Here's how the part is built. I have some questions about the finished solid (model axes, mm). A direction names the side the tool comes from. Round coordinates to 2 decimals unless told otherwise and drop trailing zeros. Order: outer loops, then holes, each group sorted by start corner. A loop starts at its lowest first (then second) coordinate and runs counter-clockwise, first axis right, second up. Notation, with made-up numbers: M 11,59.5 L 60,59.5 A27 cw 60,83.5 Z; hole C 85,-9.75 d6. An arc over 180 degrees is marked long. Write item = value, one per line. Start each with the question number.
Item 1: I want a section at D-D, the plane y = -4. List the corners of the cut face in (x, z) for me.
Item 2: We'd pull the mould along Z, two halves only. Please class faces 6 (the face through (23, -6, -13)), 7 (the face through (16.57, 6.1, 1.48)), 8 (the face through (20.76, 15.537, -7.798)): pulls with the +Z half, pulls with the -Z half, needs draft (parallel to the pull), parting line crosses it, or undercut.
Item 3: I want a section at C-C, the plane z = -8. State how many separate pieces and enclosed holes the cut face has, plus the area to 3 significant figures.
Item 4: I want a section at A-A, the plane z = -5.75. List the corners of the cut face in (x, y) for me, plus the area to 3 significant figures.
Item 5: I want a section at B-B, the plane x = 11.75. List the corners of the cut face in (y, z) for me.
Item 6: Please list where these lines run through material, in increasing order: L1, parallel to X at y = 11, z = -1; L2, parallel to Y at x = 23.35, z = -8; L3, parallel to Y at x = 25, z = -7.5.
Item 7: I'm going to push flat-ended pins straight in: P1, Ø2, axis at y = 6, z = -11.5, coming from the -X side; P2, Ø8, axis at x = 5, z = -0.5, coming from the -Y side; P3, Ø1.6, axis at x = 20.5, y = -1, coming from the +Z side; P4, Ø9.5, axis at x = 25, y = 5, coming from the -Z side. Where does each tip first touch, or does it pass through?
Item 8: For faces 1 (the face through (29.048, 5.127, -7.605)), 2 (the face through (9, 7, 0)), 3 (the face through (23, 15, -1)), 4 (the face through (23.26, 15.537, -7.798)), 5 (the face through (16.55, 3.88, 1.48)), which set-ups out of +Z, -Z, +X, -X, +Y, -Y let a thin tool reach every point of the face, with its end or its side?
```python
from build123d import *

# Parameters (mm, degrees)
SZKIC1_W                    = 30
SZKIC1_H                    = 10
DODANIE_WYCI_GNI_CIE1_DEPTH = 3
ZAOKR_GLENIE1_R             = 5
WYTNIJ_WYCI_GNI_CIE1_REACH  = 33.765
SZKIC2_W                    = 13.6
SZKIC2_H                    = 3.1
ZAOKR_GLENIE2_R             = 1.5
SZKIC3_R                    = 5
DODANIE_WYCI_GNI_CIE2_DEPTH = 15
SZKIC5_W                    = 1.5
SZKIC5_H                    = 24
DODANIE_WYCI_GNI_CIE3_DEPTH = 15
SZKIC4_R                    = 4.05
WYTNIJ_WYCI_GNI_CIE2_DEPTH  = 15
SZKIC6_W                    = 1
SZKIC6_H                    = 10.631374676
WYTNIJ_WYCI_GNI_CIE3_DEPTH  = 15
SZKIC7_R                    = 1.55
WYTNIJ_WYCI_GNI_CIE4_DEPTH  = 34.015148038
ZAOKR_GLENIE3_R             = 5
SFAZOWANIE1_SIZE            = 1


with BuildPart() as part:
    # Szkic1 → Dodanie-wyciągnięcie1 (new body)
    with BuildSketch(Plane.XY):
        with Locations((15, 5)):
            Rectangle(SZKIC1_W, SZKIC1_H)
    extrude(amount=DODANIE_WYCI_GNI_CIE1_DEPTH)

    # Zaokrąglenie1
    zaokr_glenie1_edges = [part.edges().sort_by_distance(p)[0] for p in [
        (0, 10, 1.5),
        (0, 0, 1.5),
        (30, 10, 1.5),
        (30, 0, 1.5),
    ]]
    fillet(zaokr_glenie1_edges, radius=ZAOKR_GLENIE1_R - 0.0001)  # a hair under: the kernel refuses the full size

    # Szkic2 → Wytnij-wyciągnięcie1 (cut, up to next)
    with BuildSketch(Plane.XY.offset(3), mode=Mode.PRIVATE) as wytnij_wyci_gni_cie1_sk1:
        with Locations((10.2, 5)):
            Rectangle(SZKIC2_W, SZKIC2_H)
    wytnij_wyci_gni_cie1_tool1 = extrude(wytnij_wyci_gni_cie1_sk1.sketch, amount=-WYTNIJ_WYCI_GNI_CIE1_REACH, mode=Mode.PRIVATE) & part.part
    add(wytnij_wyci_gni_cie1_tool1.solids().sort_by_distance((10.2, 5, 3))[0], mode=Mode.SUBTRACT)

    # Zaokrąglenie2
    zaokr_glenie2_edges = [part.edges().sort_by_distance(p)[0] for p in [
        (3.4, 3.45, 1.5),
        (3.4, 6.55, 1.5),
        (17, 6.55, 1.5),
        (17, 3.45, 1.5),
    ]]
    fillet(zaokr_glenie2_edges, radius=ZAOKR_GLENIE2_R)

    # Szkic3 → Dodanie-wyciągnięcie2 (add)
    with BuildSketch(Plane(origin=(0, 0, 0), x_dir=(-1, 0, 0), z_dir=(0, 0, -1))):
        with Locations((-25, 5)):
            Circle(SZKIC3_R)
    extrude(amount=DODANIE_WYCI_GNI_CIE2_DEPTH)

    # Szkic5 → Dodanie-wyciągnięcie3 (add)
    with BuildSketch(Plane(origin=(0, 0, -15), x_dir=(-1, 0, 0), z_dir=(0, 0, -1))):
        with Locations((-20.75, 5)):
            Rectangle(SZKIC5_W, SZKIC5_H)
        with Locations((-23.25, 5)):
            Rectangle(SZKIC5_W, SZKIC5_H)
    extrude(amount=-DODANIE_WYCI_GNI_CIE3_DEPTH)

    # Szkic4 → Wytnij-wyciągnięcie2 (cut)
    with BuildSketch(Plane(origin=(0, 0, -15), x_dir=(-1, 0, 0), z_dir=(0, 0, -1))):
        with Locations((-25, 5)):
            Circle(SZKIC4_R)
    extrude(amount=-WYTNIJ_WYCI_GNI_CIE2_DEPTH, mode=Mode.SUBTRACT)

    # Szkic6 → Wytnij-wyciągnięcie3 (cut)
    with BuildSketch(Plane(origin=(0, 0, -15), x_dir=(-1, 0, 0), z_dir=(0, 0, -1))):
        with Locations((-22, 4.629389041)):
            Rectangle(SZKIC6_W, SZKIC6_H)
    extrude(amount=-WYTNIJ_WYCI_GNI_CIE3_DEPTH, mode=Mode.SUBTRACT)

    # Szkic7 → Wytnij-wyciągnięcie4 (cut, through all)
    with BuildSketch(Plane(origin=(24, 0, 0), x_dir=(0, 0, -1), z_dir=(1, 0, 0))):
        with Locations((8, -4)):
            Circle(SZKIC7_R)
        with Locations((8, 14)):
            Circle(SZKIC7_R)
    extrude(amount=-WYTNIJ_WYCI_GNI_CIE4_DEPTH, mode=Mode.SUBTRACT)

    # Zaokrąglenie3
    zaokr_glenie3_edges = [part.edges().sort_by_distance(p)[0] for p in [
        (23.25, -7, -15),
        (23.25, -7, 0),
        (23.25, 17, 0),
        (23.25, 17, -15),
        (20.75, -7, -15),
        (20.75, -7, 0),
        (20.75, 17, 0),
        (20.75, 17, -15),
    ]]
    fillet(zaokr_glenie3_edges, radius=ZAOKR_GLENIE3_R)

    # Sfazowanie1
    sfazowanie1_edges = [part.edges().sort_by_distance(p)[0] for p in [
        (20, 5, 0),
    ]]
    chamfer(sfazowanie1_edges, length=SFAZOWANIE1_SIZE)


solid = part.part
```
Filled in:
q1.outline = M 20,-14.58 L 21.5,-14.58 L 21.5,-9.55 L 20,-9.55 Z; M 20,-6.45 L 21.5,-6.45 L 21.5,-0.42 L 20,-0.42 Z; M 22.5,-14.58 L 24,-14.58 L 24,-9.55 L 22.5,-9.55 Z; M 22.5,-6.45 L 24,-6.45 L 24,-0.42 L 22.5,-0.42 Z
q2.face_6 = pulls with the -Z half
q2.face_7 = needs draft
q2.face_8 = undercut
q3.separate_pieces = 6
q3.enclosed_holes = 0
q3.area = 56.4 mm^2
q4.outline = M 20,-7 L 21.5,-7 L 21.5,2.96 A4.05 cw 21.5,7.04 L 21.5,17 L 20,17 Z; M 22.5,-7 L 24,-7 L 24,0.1 A5 ccw long 24,9.9 L 24,17 L 22.5,17 L 22.5,8.19 A4.05 cw long 22.5,1.81 Z
q4.area = 75.0 mm^2
q5.outline = M 0,0 L 3.45,0 L 3.45,3 L 0,3 Z; M 6.55,0 L 10,0 L 10,3 L 6.55,3 Z
q6.L1 = 20 to 21.5, 22.5 to 24
q6.L2 = -7 to -5.55, -2.45 to 1.3, 8.7 to 12.45, 15.55 to 17
q6.L3 = 0 to 0.95, 9.05 to 10
q7.P1 = 20
q7.P2 = 0
q7.P3 = 0
q7.P4 = -15
q8.face_1 = -Z
q8.face_2 = -Z, -X, +Y, -Y
q8.face_3 = +Z, +X, -X, +Y
q8.face_4 = +X, -X
q8.face_5 = +Z, -Z
